```python
from build123d import *

# Parameters (mm, degrees)
F0_W     = 75.605
F0_H     = 56.515
F1_DEPTH = 16.8275
F2_T     = -1.5875
F3_W     = 11.938
F3_H     = 10.668
F3_W_2   = 8.73125
F4_DEPTH = 1.5875


with BuildPart() as f1:
    # F0 (on Top) → F1 (new body)
    with BuildSketch(Plane.XY):
        with Locations((15.93168, 1.055113)):
            Rectangle(F0_W, F0_H)
    extrude(amount=F1_DEPTH)

    # F2
    f2_openings = [f1.faces().sort_by_distance(p)[0] for p in [
        (15.93168, 1.055113, 16.8275),
    ]]
    offset(amount=F2_T, openings=f2_openings)

    # F3 (on face) → F4 (cut)
    with BuildSketch(Plane.YZ.offset(53.73418)):
        with Locations((-10.755887, 11.4935)):
            Rectangle(F3_W, F3_H)
        with Locations((19.562188, 11.4935)):
            Rectangle(F3_W_2, F3_H)
    extrude(amount=-F4_DEPTH, mode=Mode.SUBTRACT)


solid = f1.part
```
The listing builds one solid part. Answer for the finished solid, in the listing's coordinates (mm). A direction names the side the tool comes from. Round coordinates to 2 decimals unless told otherwise and drop trailing zeros. Loops run counter-clockwise (first coordinate to the right, second up) from the corner with the lowest first, then second, coordinate; pieces in that order, holes last. Notation, with made-up numbers: (0.5, -9.75) - (32.5, -9.75) arc R9 ccw to (32.5, 6.25) - close; hole circle Ø9 at (76, 75.25). An arc over 180 degrees is marked (long way). Return JSON: item names as keys, results as strings. Group by question number.
1. The mould has two halves that part along Y. Classify faces 4 (the flat face through (15, -27.202, 8)), 5 (the flat face through (15, 1, 0)), 6 (the flat face through (52.147, 1, 9)): pulls with the +Y half, pulls with the -Y half, needs draft (parallel to the pull), parting line crosses it, or undercut.
2. The part is cut by section A-A on z = 15. Determine the outline of the cut face in (x, y), then the cut area to 3 significant figures.
3. Which of the six approach directions +Z, -Z, +X, -X, +Y, -Y give full straight-line access (tool end or side, diameter ignored) to faces 1 (the flat face through (53, -4.787, 11)), 2 (the flat face through (15, 1, 1.588)), 3 (the flat face through (15, 29.313, 8))?
4. The part is cut by section C-C on x = -7. Determine the outline of the cut face in (y, z), then the cut area to 3 significant figures.
5. The part is cut by section B-B on y = 0.5. Determine the outline of the cut face in (x, z).
6. Consider probe 1 along Y at (x, z) = (13.5, 3); probe 2 along X at (y, z) = (-17, 2.25); probe 3 along Z at (x, y) = (-5, -1). Determine where each line is inside the solid, lowest interval first.
7. This flat-tipped pin is pushed along its axis until it touches: P1, Ø0.8, axis at x = 53, y = 18, coming from the +Z side. Where does it stop, or does it pass through?
Resolved:
{
 "1": {"face 4": "pulls with the -Y half", "face 5": "needs draft", "face 6": "undercut"},
 "2": {"outline": "(-21.87, -27.2) - (53.73, -27.2) - (53.73, -16.72) - (52.15, -16.72) - (52.15, -25.61) - (-20.28, -25.61) - (-20.28, 27.73) - (52.15, 27.73) - (52.15, 23.93) - (53.73, 23.93) - (53.73, 29.31) - (-21.87, 29.31) - close; (52.15, -4.79) - (53.73, -4.79) - (53.73, 15.2) - (52.15, 15.2) - close", "area": "377 mm²"},
 "3": {"face 1": "+Z, +X", "face 2": "+Z", "face 3": "+Z, -Z, +X, -X, +Y"},
 "4": {"outline": "(-27.2, 0) - (29.31, 0) - (29.31, 16.83) - (27.73, 16.83) - (27.73, 1.59) - (-25.61, 1.59) - (-25.61, 16.83) - (-27.2, 16.83) - close", "area": "138 mm²"},
 "5": {"outline": "(-21.87, 0) - (53.73, 0) - (53.73, 16.83) - (52.15, 16.83) - (52.15, 1.59) - (-20.28, 1.59) - (-20.28, 16.83) - (-21.87, 16.83) - close"},
 "6": {"probe 1": "y = -27.2 to -25.61, 27.73 to 29.31", "probe 2": "x = -21.87 to -20.28, 52.15 to 53.73", "probe 3": "z = 0 to 1.59"},
 "7": {"P1": "stops at z = 6.16"}
}
